Work out the finished part from the listing and answer in its coordinate system (mm). A direction names the side the tool comes from. Coordinates: 2 decimals unless noted, no trailing zeros. Loops run counter-clockwise (first coordinate to the right, second up) from the corner with the lowest first, then second, coordinate; pieces in that order, holes last. Notation, with made-up numbers: (41, 57) -> (64, 57) arc R20 cw to (64, 76) -> close; hole circle Ø1 at (-5, 58.25). An arc over 180 degrees is marked (long way). One line per question, with ' | ' between items.
Autodesk Inventor part; units mm, degrees
ref_plane "Work Plane1" through (124.725, 49.8, -24.875) normal (0, 1, 0) x (0, 0, 1)
ref_plane "YZ Plane" through (0, 0, 0) normal (1, 0, 0) x (0, 1, 0)
ref_plane "XZ Plane" through (0, 0, 0) normal (0, 1, 0) x (-1, 0, 0)
sketch "Sketch1" plane through (0, 0, 0) normal (0, 1, 0) x (-1, 0, 0)
  line L0 (-155.225, -15) -> (-155.225, 15)
  line L1 (-155.225, 15) -> (-147.725, 15)
  line L2 (-147.725, 15) -> (-147.725, -15)
  line L3 (-147.725, -15) -> (-155.225, -15)
  circle A0 centre (-171.5, -21.9) radius 1.875
  circle A1 centre (-127.7, 21.9) radius 1.875
  circle A2 centre (-127.7, -21.9) radius 1.875
  circle A3 centre (-171.5, 21.9) radius 1.875
  circle A4 centre (-135.2, 20.8) radius 2.0734
  circle A5 centre (-164, -20.8) radius 2.0734
  circle A6 centre (-135.2, -20.8) radius 2.0734
  circle A7 centre (-128.8, -14.4) radius 2.0734
  circle A8 centre (-128.8, 14.4) radius 2.0734
  circle A9 centre (-164, 20.8) radius 2.0734
  circle A10 centre (-170.4, -14.4) radius 2.0734
  circle A11 centre (-170.4, 14.4) radius 2.0734
  line L4 (-172.5, 24.875) -> (-126.7, 24.875)
  arc A12 (-172.5, 24.875) -> (-174.475, 22.9) centre (-172.5, 22.9) ccw
  line L5 (-174.475, -22.9) -> (-174.475, 22.9)
  arc A13 (-174.475, -22.9) -> (-172.5, -24.875) centre (-172.5, -22.9) ccw
  line L6 (-126.7, -24.875) -> (-172.5, -24.875)
  arc A14 (-126.7, -24.875) -> (-124.725, -22.9) centre (-126.7, -22.9) ccw
  line L7 (-124.725, 22.9) -> (-124.725, -22.9)
  arc A15 (-124.725, 22.9) -> (-126.7, 24.875) centre (-126.7, 22.9) ccw
  point P0 (0, 0)
ref_plane "Work Plane1" through (124.725, 49.8, -24.875) normal (0, 1, 0) x (0, 0, 1)
extrude "Extrusion1" add sketch "Sketch1" along normal blind 4 from surface at 49.8 contours A0 | A1 | A2 | A3 | L4 A15 L7 A14 L6 A13 L5 A12
sketch "Sketch2" plane through (126.7, 53.8, -24.875) normal (0, 1, 0) x (1, 0, 0)
  line L0 (28.525, -9.875) -> (21.025, -9.875)
  line L1 (28.525, -39.875) -> (28.525, -9.875)
  line L2 (21.025, -39.875) -> (28.525, -39.875)
  line L3 (21.025, -9.875) -> (21.025, -39.875)
  circle A0 centre (8.5, -45.675) radius 2.0734
  circle A1 centre (37.3, -4.075) radius 2.0734
  circle A2 centre (8.5, -4.075) radius 2.0734
  circle A3 centre (2.1, -10.475) radius 2.0734
  circle A4 centre (2.1, -39.275) radius 2.0734
  circle A5 centre (37.3, -45.675) radius 2.0734
  circle A6 centre (43.7, -10.475) radius 2.0734
  circle A7 centre (43.7, -39.275) radius 2.0734
  arc A8 (47.775, -1.975) -> (45.8, 0) centre (45.8, -1.975) ccw
  line L4 (0, 0) -> (45.8, 0)
  arc A9 (0, 0) -> (-1.975, -1.975) centre (0, -1.975) ccw
  line L5 (-1.975, -47.775) -> (-1.975, -1.975)
  arc A10 (-1.975, -47.775) -> (0, -49.75) centre (0, -47.775) ccw
  line L6 (45.8, -49.75) -> (0, -49.75)
  arc A11 (45.8, -49.75) -> (47.775, -47.775) centre (45.8, -47.775) ccw
  line L7 (47.775, -1.975) -> (47.775, -47.775)
  line L8 (18.525, -42.375) -> (31.025, -42.375)
  line L9 (31.025, -42.375) -> (31.025, -7.375)
  line L10 (31.025, -7.375) -> (18.525, -7.375)
  line L11 (18.525, -7.375) -> (18.525, -42.375)
  line L12 (45.8, 0) -> (52.05, 0)
  line L13 (52.05, 0) -> (52.05, -49.75)
  line L14 (52.05, -49.75) -> (45.8, -49.75)
  line L15 (45.8, -49.75) -> (45.8, 0)
  line L16 (52.05, -49.75) -> (47.925, -49.75)
  line L17 (47.925, -49.75) -> (47.925, 0)
  line L18 (47.925, 0) -> (52.05, 0)
  line L19 (52.05, 0) -> (52.05, -49.75)
  arc A12 (45.8, -49.875) -> (47.9, -47.775) centre (45.8, -47.775) ccw
  line L20 (45.8, -49.875) -> (0, -49.875)
  arc A13 (-2.1, -47.775) -> (0, -49.875) centre (0, -47.775) ccw
  line L21 (-2.1, -47.775) -> (-2.1, -1.975)
  arc A14 (0, 0.125) -> (-2.1, -1.975) centre (0, -1.975) ccw
  line L22 (0, 0.125) -> (45.8, 0.125)
  arc A15 (47.9, -1.975) -> (45.8, 0.125) centre (45.8, -1.975) ccw
  line L23 (47.9, -1.975) -> (47.9, -47.775)
  line L24 (18.525, -42.375) -> (11.025, -42.375)
  line L25 (11.025, -42.375) -> (11.025, -7.375)
  line L26 (11.025, -7.375) -> (18.525, -7.375)
  line L27 (18.525, -7.375) -> (18.525, -42.375)
  line L28 (31.025, -42.375) -> (38.525, -42.375)
  line L29 (38.525, -42.375) -> (38.525, -7.375)
  line L30 (38.525, -7.375) -> (31.025, -7.375)
  line L31 (31.025, -7.375) -> (31.025, -42.375)
  point P0 (-126.7, -24.875)
  point P1 (46.5137, -49.75)
  point P2 (46.5137, 0)
  point P3 (31.025, -7.375)
  point P4 (18.525, -7.375)
  dimension "d2" = 2.5
  dimension "d3" = 6.25
  dimension "d4" = 4.125
  dimension "d15" = 0.125
  dimension "d16" = 7.5
  dimension "d17" = 7.5
extrude "Extrusion2" cut sketch "Sketch2" against normal up to surface (4 mm away) contours L11 L10 L9 L8
extrude "Extrusion3" add sketch "Sketch2" against normal up to surface (4 mm away) contours A8 L12 A15 L23 A12 L14 A11 L7 | L12 L17 L14 A12 L23 A15 | L12 L13 L14 L17
extrude "Extrusion4" add sketch "Sketch2" against normal blind 49.8 from surface at -4 contours L12 L17 L14 A12 L23 A15 | L12 L13 L14 L17
extrude "Extrusion5" cut sketch "Sketch2" along normal blind 2 from surface at -4 contours L24 L25 L26 L11 | L9 L30 L29 L28
fillet "Fillet1" radius 2 2 edges at (178.75, 26.9, 24.875) (178.75, 26.9, -24.875)
sketch "Sketch3" plane through (178.75, 53.8, 22.875) normal (1, 0, 0) x (0, 0, -1)
  line L0 (7.875, -23.425) -> (7.875, -30.925)
  line L1 (7.875, -30.925) -> (37.875, -30.925)
  line L2 (37.875, -30.925) -> (37.875, -23.425)
  line L3 (37.875, -23.425) -> (7.875, -23.425)
  line L4 (5.825, -11.7) -> (39.925, -11.7)
  line L5 (39.925, -46.1) -> (39.925, -11.7)
  line L6 (5.825, -46.1) -> (39.925, -46.1)
  line L7 (5.825, -11.7) -> (5.825, -46.1)
  line L8 (5.375, -20.925) -> (5.375, -33.425)
  line L9 (5.375, -33.425) -> (40.375, -33.425)
  line L10 (40.375, -33.425) -> (40.375, -20.925)
  line L11 (40.375, -20.925) -> (5.375, -20.925)
  point P0 (22.875, -53.8)
  point P1 (39.925, -20.925)
  point P2 (5.825, -20.925)
  point P3 (5.825, -33.425)
  point P4 (39.925, -33.425)
  dimension "d12" = 2.5
extrude "Extrusion6" cut sketch "Sketch3" against normal up to surface (4.15 mm away) contours L3 L2 L1 L0 | L11 L5 L9 L7
sketch "Sketch4" plane through (178.75, 53.8, 22.875) normal (1, 0, 0) x (0, 0, -1)
  line L0 (5.825, -20.925) -> (39.925, -20.925)
  line L1 (39.925, -20.925) -> (39.925, -33.425)
  line L2 (39.925, -33.425) -> (5.825, -33.425)
  line L3 (5.825, -33.425) -> (5.825, -20.925)
  line L4 (45.75, 0) -> (45.75, -53.8)
  line L5 (0, 0) -> (45.75, 0)
  line L6 (0, -53.8) -> (0, 0)
  line L7 (45.75, -53.8) -> (0, -53.8)
  line L8 (5.825, -20.925) -> (39.925, -20.925)
  line L9 (39.925, -20.925) -> (39.925, -13.425)
  line L10 (39.925, -13.425) -> (5.825, -13.425)
  line L11 (5.825, -13.425) -> (5.825, -20.925)
  line L12 (5.825, -33.425) -> (39.925, -33.425)
  line L13 (39.925, -33.425) -> (39.925, -40.925)
  line L14 (39.925, -40.925) -> (5.825, -40.925)
  line L15 (5.825, -40.925) -> (5.825, -33.425)
  point P0 (22.875, -53.8)
  point P1 (39.925, -20.925)
  dimension "d20" = 7.5
  dimension "d21" = 7.5
extrude "Extrusion7" cut sketch "Sketch4" along normal blind 2 from surface at -4.15 contours L11 L10 L9 L0 | L2 L13 L14 L15
chamfer "Chamfer1" distance 2 angle 45 2 edges at (174.6, 40.375, 0) (174.6, 12.875, 0)
properties part number "Lens Light Cover"
1) Find section D-D (y = 6.5). Write down the section's boundary in (x, z) (3 decimals).
Check values:
outline: (173.214, -24.875) -> (176.75, -24.875) arc R2 ccw to (178.75, -22.875) -> (178.75, 22.875) arc R2 ccw to (176.75, 24.875) -> (173.214, 24.875) arc R2.1 cw to (174.6, 22.9) -> (174.6, -22.9) arc R2.1 cw to start
2) For faces 4 (the face through (157.725, 53, 0)), 5 (the face through (178, 20.375, 0)), 6 (the face through (176.6, 17, 0)), 7 (the face through (151, 51, -17.5)), determine the directions among +Z, -Z, +X, -X, +Y, -Y from which every point of the face is accessible in a straight line to the end or side of a thin tool.
Check values:
face 4: +Y, -Y | face 5: +X, -X | face 6: -X | face 7: -Y
3) The mould has two halves that part along Z. Classify faces 1 (the face through (176.6, 37, 0)), 2 (the face through (177, 0, 0)), 3 (the face through (174, 39, 24.875)): released by +Z, released by -Z, zero draft, split by the parting line, or undercut.
Check values:
face 1: undercut | face 2: zero draft | face 3: released by +Z
4) Flat-ended cylindrical pins translate along their axes: pin 1 (10 mm diameter, centred on x = 140.5, z = 9, fed in from -Y); pin 2 (13.5 mm diameter, centred on y = 35.5, z = 9, fed in from -X); pin 3 (6 mm diameter, centred on y = 39.5, z = 18, fed in from -X). Find the tip coordinate at first contact, or state that the pin passes through.
Check values:
pin 1: stops at y = 49.8 | pin 2: stops at x = 174.72 | pin 3: stops at x = 174.6
5) Find section A-A (z = 9). State how many separate pieces and enclosed holes the cut face has, plus the area to 3 significant figures.
Check values:
separate pieces: 3 | enclosed holes: 0 | area: 257 mm^2
6) Find section B-B (x = 170.4). Write down the section's boundary in (y, z) (3 decimals), plus the area to 3 significant figures.
Check values:
outline: (49.8, -24.875) -> (53.8, -24.875) -> (53.8, -16.473) -> (49.8, -16.473) -> close; (49.8, -12.327) -> (53.8, -12.327) -> (53.8, 12.327) -> (49.8, 12.327) -> close; (49.8, 16.473) -> (53.8, 16.473) -> (53.8, 24.875) -> (49.8, 24.875) -> close | area: 166 mm^2
7) Find the intervals of material crossed by line 1 along Z through (x, y) = (170.4, 52.1) (3 decimals); line 2 along Z through (x, y) = (164, 51) (3 decimals); line 3 along Z through (x, y) = (135.2, 51) (3 decimals), in increasing order.
Check values:
line 1: z = -24.875 to -16.473, -12.327 to 12.327, 16.473 to 24.875 | line 2: z = -24.875 to -22.873, -18.727 to -17.5, 17.5 to 18.727, 22.873 to 24.875 | line 3: z = -24.875 to -22.873, -18.727 to 18.727, 22.873 to 24.875
